Autodesk Fusion 360 part; units mm, degrees
sketch "Sketch1" plane through (0, 0, 0) normal (0, 0, 1) x (1, 0, 0)
  line L0 (0, 0) -> (160, 0)
  circle A0 centre (0, 0) radius 3
  circle A1 centre (160, 0) radius 3
  circle A2 centre (0, 0) radius 9
  circle A3 centre (160, 0) radius 9
  line L1 (-9, 9) -> (169, 9)
  line L2 (169, 9) -> (169, -9)
  line L3 (169, -9) -> (-9, -9)
  line L4 (-9, -9) -> (-9, 9)
  line L5 (-3, 9) -> (3, 9)
  line L6 (3, 9) -> (3, -3)
  line L7 (3, -3) -> (-3, -3)
  line L8 (-3, -3) -> (-3, 9)
  line L9 (157, 3) -> (163, 3)
  line L10 (163, 3) -> (163, -9)
  line L11 (163, -9) -> (157, -9)
  line L12 (157, -9) -> (157, 3)
  dimension "d1" = 160
  dimension "d2" = 6
  dimension "d3" = 6
  dimension "d4" = 18
  dimension "d5" = 18
extrude "Extrude1" add sketch "Sketch1" along normal blind 4 contours L0 A2 L6 | A0 L6 L7 | L0 A2 L6 L7 L8 | L0 A2 A3 L1 L6 | L0 A2 A3 L3 L12 | A0 L7 L8 | L0 A3 L9 L10 L12 | L0 A3 L12 | A2 L1 L4 L8 | A1 L9 L12 | A1 L9 L10 | A3 L2 L3 L10
fillet "Fillet1" radius 5 2 edges at (157, -9, 2) (3, 9, 2)
Design review of the part built by this model. Coordinates are the model's own, in mm. A direction names the side the tool comes from. Coordinates: 2 decimals unless noted, no trailing zeros. Order: outer loops, then holes, each group sorted by start corner. A loop starts at its lowest first (then second) coordinate and runs counter-clockwise, first axis right, second up.
Item 1: For faces 1 (the cylindrical face through (-6.294, -6.434, 1.972)), 2 (the cylindrical face through (155, -8, 2)), 3 (the flat face through (-3, 4, 2)), list the 3-axis set-ups (+Z, -Z, +X, -X, +Y, -Y) from which the entire face can be reached by the end or side of a thin tool; tool diameter is ignored.
Item 2: The part is to be moulded in two halves that separate along X. For faces 4 (the flat face through (163, -4, 2)), 5 (the flat face through (166, -9, 2)), 6 (the flat face through (169, -4, 2)), say which applies: pulls with the +X half, pulls with the -X half, needs draft (parallel to the pull), parting line crosses it, or undercut.
Item 3: For pin 1 Ø2 at (y, z) = (3.5, 1.5) entering from +X; pin 2 Ø1.2 at (y, z) = (-3, 2) entering from -X, all flat-tipped, find the tip position at first contact; note any pin that passes through.
Item 4: For line 1 (X direction, y = 0, z = 0.4); line 2 (X direction, y = 1, z = 1.1); line 3 (X direction, y = 6.75, z = 3.75), list the stretches that pass through material, from the lowest coordinate up.
Item 5: Take a section at A-A, the plane z = 1.4. Write out the cut boundary in (x, y).
The answers:
1. face 1: +Z, -Z, -X, -Y
1. face 2: +Z, -Z, -Y
1. face 3: +Z, -Z, +Y
2. face 4: undercut
2. face 5: needs draft
2. face 6: pulls with the +X half
3. pin 1: stops at x = 168.65
3. pin 2: stops at x = -8.67
4. line 1: x = -9 to -3, 3 to 157, 163 to 169
4. line 2: x = -9 to -3, 3 to 157.17, 162.83 to 168.94
4. line 3: x = -9 to -3, 3.82 to 165.95
5. outline: (-9, 0) arc R9 ccw to (0, -9) - (152, -9) arc R5 ccw to (157, -4) - (157, 0) arc R3 cw to (163, 0) - (163, -9) - (169, -9) - (169, 0) arc R9 ccw to (160, 9) - (8, 9) arc R5 ccw to (3, 4) - (3, 0) arc R3 cw to (-3, 0) - (-3, 9) - (-9, 9) - close
